from build123d import *

# Parameters (mm, degrees)
F1_DEPTH = 1.9


with BuildPart() as f1:
    # F0 (on Front) → F1 (new body)
    with BuildSketch(Plane.XZ):
        with BuildLine():
            ThreePointArc((-1.258524, -0.325757), (0.201208, 1.284335), (1.098604, -0.695032))
            Line((1.098604, -0.695032), (1.466869, -0.928015))
            ThreePointArc((1.466869, -0.928015), (1.667194, -0.483095), (1.735775, 0))
            Line((1.735775, 0), (16.358244, 0))
            ThreePointArc((16.358244, 0), (16.426825, -0.483095), (16.62715, -0.928015))
            Line((16.62715, -0.928015), (16.995415, -0.695032))
            ThreePointArc((16.995415, -0.695032), (17.892811, 1.284335), (19.352543, -0.325757))
            Line((19.352543, -0.325757), (19.774415, -0.434954))
            ThreePointArc((19.774415, -0.434954), (18.960684, 1.503931), (16.875129, 1.235808))
            Line((16.875129, 1.235808), (1.479197, 0.908235))
            ThreePointArc((1.479197, 0.908235), (-0.679087, 1.597422), (-1.680396, -0.434954))
            Line((-1.680396, -0.434954), (-1.258524, -0.325757))
        make_face()
        Polygon((1.727705, 0.330091), (1.704895, 0.626613), (16.394122, 0.866111), (16.268671, 0.330091), align=None, mode=Mode.SUBTRACT)
    extrude(amount=F1_DEPTH)


solid = f1.part
CAD build for the part. Positions are in the model's coordinates, mm. A direction names the side the tool comes from. Round coordinates to 2 decimals unless told otherwise and drop trailing zeros. Loops run counter-clockwise (first coordinate to the right, second up) from the corner with the lowest first, then second, coordinate; pieces in that order, holes last. Notation, with made-up numbers: M 59,8.25 L 114,8.25 A24 cw 114,19.25 Z; hole C 83,61 d7. An arc over 180 degrees is marked long. One line per question, with ' | ' between items. Start each with the question number.
Item 1: Pin check, flat tips, straight feed: pin 1 Ø1 at (x, y) = (2, -0.5) entering from -Z; pin 2 Ø0.6 at (x, y) = (7, -0.5) entering from -Z. Stop position of each tip, or through.
Item 2: Cut at A-A, the plane y = -1.3. Write the cut outline in (x, z).
Item 3: Cut at B-B, the plane x = 16. Write the cut outline in (y, z).
Item 4: Two-plate mould, pull along X, no slides. Class faces 4 (the cylindrical face through (1.665, -0.937, -0.49)), 5 (the flat face through (9, 0, 0.9)): pulls with the +X half, pulls with the -X half, needs draft (parallel to the pull), parting line crosses it, or undercut.
Item 5: Wall check: line 1 (Z direction, x = 18, y = -0.1); line 2 (X direction, y = -1.6, z = -0.2); line 3 (Z direction, x = 11, y = -0.45). Give the ranges that are in metal, low to high.
Item 6: Cut at C-C, the plane x = 0. Write the cut outline in (y, z), plus the area to 3 significant figures.
Item 7: Which spindle directions (+Z, -Z, +X, -X, +Y, -Y) get a long thin tool onto all of the face, cutting with end or side? Do faces 1 (the flat face through (9, -1.9, 0.9)), 2 (the flat face through (9, -1, 0.33)), 3 (the cylindrical face through (16.425, -0.937, -0.477)). Say none if no direction does.
Responses:
1) pin 1: stops at z = -0.87 | pin 2: stops at z = 0
2) outline: M -1.68,-0.43 L -1.26,-0.33 A1.3 cw long 1.1,-0.7 L 1.47,-0.93 A1.74 ccw 1.74,0 L 16.36,0 A1.74 ccw 16.63,-0.93 L 17,-0.7 A1.3 cw long 19.35,-0.33 L 19.77,-0.43 A1.74 ccw 16.88,1.24 L 1.48,0.91 A1.74 ccw Z; hole M 1.7,0.63 L 1.73,0.33 L 16.27,0.33 L 16.39,0.87 Z
3) outline: M -1.9,0 L 0,0 L 0,0.33 L -1.9,0.33 Z; M -1.9,0.86 L 0,0.86 L 0,1.22 L -1.9,1.22 Z
4) face 4: undercut | face 5: needs draft
5) line 1: z = 1.3 to 1.73 | line 2: x = -1.72 to -1.28, 1.28 to 1.72, 16.37 to 16.81, 19.38 to 19.82 | line 3: z = 0 to 0.33, 0.78 to 1.11
6) outline: M -1.9,1.3 L 0,1.3 L 0,1.74 L -1.9,1.74 Z | area: 0.828 mm²
7) face 1: +Z, -Z, +X, -X, -Y | face 2: +Y, -Y | face 3: -Z, +Y, -Y
